```python
from build123d import *

# Parameters (mm, degrees)
SKETCH_1_W         = 1200
SKETCH_1_H         = 2000
EXTRUDE_1_DEPTH    = 50
SKETCH_2_W         = 25
SKETCH_2_H         = 50
EXTRUDE_2_DEPTH    = 320
EXTRUDE_1_2_DEPTH  = 35
SKETCH_4_W         = 1200
SKETCH_4_H         = 20
EXTRUDE_3_DEPTH    = 35
MIRROR_START       = -1000
MIRROR_2_OUTLINE_W = 1200
MIRROR_2_OUTLINE_H = 20
MIRROR_2_DEPTH     = 2000
MIRROR_START_2     = -1035
MIRROR_2_2_DEPTH   = 35


# Read off the part's stored shape, not the designer's step: 镜向2
with BuildPart() as part:
    # 草图1 → Extrude 1 (new body)
    with BuildSketch(Plane(origin=(0, 0, 0), x_dir=(1, 0, 0), z_dir=(0, 1, 0))):
        Rectangle(SKETCH_1_W, SKETCH_1_H)
    extrude(amount=-EXTRUDE_1_DEPTH)

    # 草图2 → 凸台-拉伸2 (add)
    with BuildSketch(Plane(origin=(0, 0, 0), x_dir=(1, 0, 0), z_dir=(0, 1, 0))):
        with Locations((-587.5, 0)):
            Rectangle(SKETCH_2_W, SKETCH_2_H)
    extrude_2 = extrude(amount=-EXTRUDE_2_DEPTH)

    # 镜向1: 凸台-拉伸2 across plane
    add(extrude_2.mirror(Plane(origin=(0, 0, 0), x_dir=(0, 0, 1), z_dir=(1, 0, 0))))

    # 草图3 → Extrude 1 2 (add)
    with BuildSketch(Plane.XY.offset(1000)):
        with BuildLine():
            Line((-600, -320), (-600, 80))
            ThreePointArc((-600, 80), (-570.710678119, 150.710678119), (-500, 180))
            Line((-500, 180), (-363.0422981, 180))
            ThreePointArc((-363.0422981, 180), (-255.876535707, 185.885952353), (-150, 203.473000167))
            ThreePointArc((-150, 203.473000167), (0, 220), (150, 203.473000167))
            ThreePointArc((150, 203.473000167), (255.876535707, 185.885952353), (363.0422981, 180))
            Line((363.0422981, 180), (500, 180))
            ThreePointArc((500, 180), (570.710678119, 150.710678119), (600, 80))
            Line((600, 80), (600, -320))
            Line((600, -320), (580, -320))
            Line((580, -320), (580, 80))
            ThreePointArc((580, 80), (556.568542495, 136.568542495), (500, 160))
            Line((500, 160), (363.0422981, 160))
            ThreePointArc((363.0422981, 160), (253.686190615, 166.006254459), (145.645660129, 183.952761329))
            ThreePointArc((145.645660129, 183.952761329), (0, 200), (-145.645660129, 183.952761329))
            ThreePointArc((-145.645660129, 183.952761329), (-253.686190615, 166.006254459), (-363.0422981, 160))
            Line((-363.0422981, 160), (-500, 160))
            ThreePointArc((-500, 160), (-556.568542495, 136.568542495), (-580, 80))
            Line((-580, 80), (-580, -320))
            Line((-580, -320), (-600, -320))
        make_face()
    extrude(amount=EXTRUDE_1_2_DEPTH)

    # 草图4 → 拉伸-薄壁3 (add)
    with BuildSketch(Plane.XY.offset(1000)):
        with Locations((0, -110)):
            Rectangle(SKETCH_4_W, SKETCH_4_H)
    extrude(amount=EXTRUDE_3_DEPTH)

    # 镜向2 outline → 镜向2 (add)
    with BuildSketch(Plane.XY.offset(MIRROR_START)):
        with Locations((0, -110)):
            Rectangle(MIRROR_2_OUTLINE_W, MIRROR_2_OUTLINE_H)
    extrude(amount=MIRROR_2_DEPTH)

    # Mirror 2 2 outline → Mirror 2 2 (add)
    with BuildSketch(Plane.XY.offset(MIRROR_START_2)):
        with BuildLine():
            ThreePointArc((-580, 80), (-556.568542495, 136.568542495), (-500, 160))
            Line((-500, 160), (-363.0422981, 160))
            ThreePointArc((-363.0422981, 160), (-253.686190616, 166.006254459), (-145.645660129, 183.952761329))
            ThreePointArc((-145.645660129, 183.952761329), (0, 200), (145.645660129, 183.952761329))
            ThreePointArc((145.645660129, 183.952761329), (253.686190616, 166.006254459), (363.0422981, 160))
            Line((363.0422981, 160), (500, 160))
            ThreePointArc((500, 160), (556.568542495, 136.568542495), (580, 80))
            Line((580, 80), (580, -320))
            Line((580, -320), (600, -320))
            Line((600, -320), (600, 80))
            ThreePointArc((600, 80), (570.710678119, 150.710678119), (500, 180))
            Line((500, 180), (363.0422981, 180))
            ThreePointArc((363.0422981, 180), (255.876535708, 185.885952353), (150, 203.473000167))
            ThreePointArc((150, 203.473000167), (0, 220), (-150, 203.473000167))
            ThreePointArc((-150, 203.473000167), (-255.876535708, 185.885952353), (-363.0422981, 180))
            Line((-363.0422981, 180), (-500, 180))
            ThreePointArc((-500, 180), (-570.710678119, 150.710678119), (-600, 80))
            Line((-600, 80), (-600, -320))
            Line((-600, -320), (-580, -320))
            Line((-580, -320), (-580, 80))
        make_face()
    extrude(amount=MIRROR_2_2_DEPTH)


solid = part.part
```
Check sheet for the modelled part. Datum: model origin and axes. Units: mm. A direction names the side the tool comes from. Round coordinates to 2 decimals unless told otherwise and drop trailing zeros. Loops run counter-clockwise (first coordinate to the right, second up) from the corner with the lowest first, then second, coordinate; pieces in that order, holes last. Notation, with made-up numbers: (41, 19.5) -> (72, 19.5) arc R17 ccw to (72, 31.5) -> close; hole circle Ø9 at (84, 76.25). An arc over 180 degrees is marked (long way). Answer in a Markdown table with one row per item.
Q1. Release check for a two-part mould opening along X. For faces 5 (the face through (571.484, 149.929, -1017.745)), 6 (the face through (555.94, 137.19, -1017.74)), 7 (the face through (-92, 200, -1000)) record: released by +X, released by -X, zero draft, split by the parting line, or undercut.
Data:
| item | result |
|---|---|
| face 5 | released by +X |
| face 6 | undercut |
| face 7 | zero draft |
Q2. Go/stop test with flat-tipped pins: P1, Ø3, axis at x = 294.5, z = 41.5, coming from the +Y side; P2, Ø17.5, axis at x = 459.5, z = -1015, coming from the +Y side; P3, Ø12, axis at x = -64.5, y = -49, coming from the -Z side. Record where each tip stops, or that it passes through.
Data:
| item | result |
|---|---|
| P1 | stops at y = 0 |
| P2 | stops at y = 180 |
| P3 | stops at z = -1000 |
Q3. Sectioned sample at A-A on y = -215.5. Enter the section's corners in (x, z), then the cut area to 3 significant figures.
Data:
| item | result |
|---|---|
| outline | (-600, -1035) -> (-580, -1035) -> (-580, -1000) -> (-600, -1000) -> close; (-600, -25) -> (-575, -25) -> (-575, 25) -> (-600, 25) -> close; (-600, 1000) -> (-580, 1000) -> (-580, 1035) -> (-600, 1035) -> close; (575, -25) -> (600, -25) -> (600, 25) -> (575, 25) -> close; (580, -1035) -> (600, -1035) -> (600, -1000) -> (580, -1000) -> close; (580, 1000) -> (600, 1000) -> (600, 1035) -> (580, 1035) -> close |
| area | 5,300 mm^2 |
Q4. Sectioned sample at C-C on x = -72.5. Enter the section's corners in (y, z), then the cut area to 3 significant figures.
Data:
| item | result |
|---|---|
| outline | (-120, -1000) -> (-100, -1000) -> (-100, 1035) -> (-120, 1035) -> close; (-50, -1000) -> (0, -1000) -> (0, 1000) -> (-50, 1000) -> close; (196.06, -1035) -> (216.17, -1035) -> (216.17, -1000) -> (196.06, -1000) -> close; (196.06, 1000) -> (216.17, 1000) -> (216.17, 1035) -> (196.06, 1035) -> close |
| area | 142,000 mm^2 |
Q5. Set-up check for faces 1 (the face through (-8, -25, -1000)), 2 (the face through (-575, -219, 0)), 3 (the face through (136, -109, 1035)), 4 (the face through (-575, -75, 0)): record each of +Z, -Z, +X, -X, +Y, -Y from which the full face is reachable in a straight line by a thin tool's end or side.
Data:
| item | result |
|---|---|
| face 1 | -Z, -Y |
| face 2 | +Z, -Z, -Y |
| face 3 | +Z, +X, -X, +Y, -Y |
| face 4 | +Z, -Z |
Q6. Sectioned sample at D-D on y = 113.5. Enter the section's corners in (x, z), then the cut area to 3 significant figures.
Data:
| item | result |
|---|---|
| outline | (-594.22, -1035) -> (-572.65, -1035) -> (-572.65, -1000) -> (-594.22, -1000) -> close; (-594.22, 1000) -> (-572.65, 1000) -> (-572.65, 1035) -> (-594.22, 1035) -> close; (572.65, -1035) -> (594.22, -1035) -> (594.22, -1000) -> (572.65, -1000) -> close; (572.65, 1000) -> (594.22, 1000) -> (594.22, 1035) -> (572.65, 1035) -> close |
| area | 3,020 mm^2 |
Q7. Sectioned sample at B-B on z = 292.5. Enter the section's corners in (x, y).
Data:
| item | result |
|---|---|
| outline | (-600, -120) -> (600, -120) -> (600, -100) -> (-600, -100) -> close; (-600, -50) -> (600, -50) -> (600, 0) -> (-600, 0) -> close |
Q8. Thickness scan on L1, parallel to Y at x = -103.5, z = -703; L2, parallel to Z at x = 363, y = -103. Record the ranges inside material, lowest first.
Data:
| item | result |
|---|---|
| L1 | y = -120 to -100, -50 to 0 |
| L2 | z = -1000 to 1035 |
